```python
from build123d import *

# Parameters (mm, degrees)
SKETCH1_R           = 49
SKETCH1_R_2         = 14.5
SKETCH1_R_3         = 3.25
BOSS_EXTRUDE1_DEPTH = 1.4


with BuildPart() as part:
    # Sketch1 → Boss-Extrude1 (new body, symmetric)
    with BuildSketch(Plane(origin=(0, 0, 0), x_dir=(1, 0, 0), z_dir=(0, 1, 0))):
        Circle(SKETCH1_R)
        Circle(SKETCH1_R_2, mode=Mode.SUBTRACT)
        with Locations((0, 19.75)):
            Circle(SKETCH1_R_3, mode=Mode.SUBTRACT)
        with Locations((19.75, 0)):
            Circle(SKETCH1_R_3, mode=Mode.SUBTRACT)
        with Locations((0, -19.75)):
            Circle(SKETCH1_R_3, mode=Mode.SUBTRACT)
        with Locations((-19.75, 0)):
            Circle(SKETCH1_R_3, mode=Mode.SUBTRACT)
    extrude(amount=BOSS_EXTRUDE1_DEPTH, both=True)


solid = part.part
```
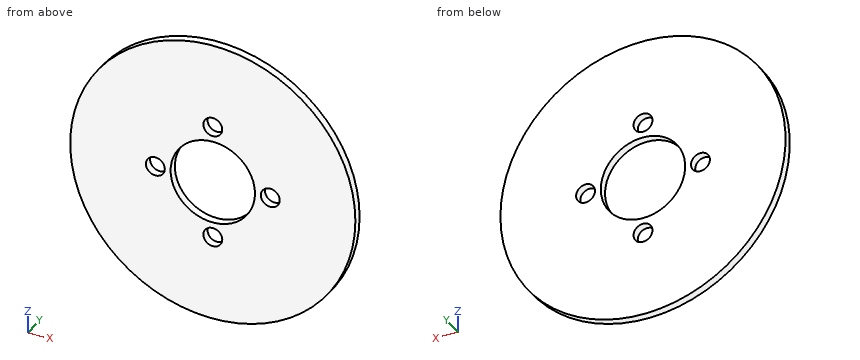
Geometry: final body of the model. Coordinates: model frame, mm. Round coordinates to 2 decimals unless told otherwise and drop trailing zeros. Write each loop counter-clockwise with the first axis right and the second up, starting at its lowest first coordinate (ties: lowest second). Pieces come first, ordered by that corner, then holes.
Item 1: Section query B-B (x = -19.75). Return loops of the section in (y, z), plus the area to 3 significant figures.
Item 2: Pin query (flat end, axial travel): P1, Ø8.5, axis at x = -19.75, z = 0, coming from the -Y side; P2, Ø4, axis at x = -35, z = -38, coming from the -Y side; P3, Ø1, axis at x = 20.5, y = 0.5, coming from the +Z side. Return the tip coordinate at first contact, or that it passes through.
Item 3: Section query C-C (y = 0.3). Return loops of the section in (x, z).
Item 4: Section query D-D (z = -19.75). Return loops of the section in (x, y), plus the area to 3 significant figures.
Item 5: Section query A-A (z = 0). Return loops of the section in (x, y), plus the area to 3 significant figures.
Item 6: Material intervals for L1, parallel to Z at x = 0, y = -0.8; L2, parallel to Z at x = 7.5, y = 0.95, sorted ascending.
Completed:
1. outline: (-1.4, -44.84) - (1.4, -44.84) - (1.4, -3.25) - (-1.4, -3.25) - close; (-1.4, 3.25) - (1.4, 3.25) - (1.4, 44.84) - (-1.4, 44.84) - close
1. area: 233 mm2
2. P1: stops at y = -1.4
2. P2: passes through
2. P3: stops at z = 44.73
3. outline: circle Ø98 at (0, 0); hole circle Ø6.5 at (-19.75, 0); hole circle Ø29 at (0, 0); hole circle Ø6.5 at (0, -19.75); hole circle Ø6.5 at (0, 19.75); hole circle Ø6.5 at (19.75, 0)
4. outline: (-44.84, -1.4) - (-3.25, -1.4) - (-3.25, 1.4) - (-44.84, 1.4) - close; (3.25, -1.4) - (44.84, -1.4) - (44.84, 1.4) - (3.25, 1.4) - close
4. area: 233 mm2
5. outline: (-49, -1.4) - (-23, -1.4) - (-23, 1.4) - (-49, 1.4) - close; (-16.5, -1.4) - (-14.5, -1.4) - (-14.5, 1.4) - (-16.5, 1.4) - close; (14.5, -1.4) - (16.5, -1.4) - (16.5, 1.4) - (14.5, 1.4) - close; (23, -1.4) - (49, -1.4) - (49, 1.4) - (23, 1.4) - close
5. area: 157 mm2
6. L1: z = -49 to -23, -16.5 to -14.5, 14.5 to 16.5, 23 to 49
6. L2: z = -48.42 to -12.41, 12.41 to 48.42
